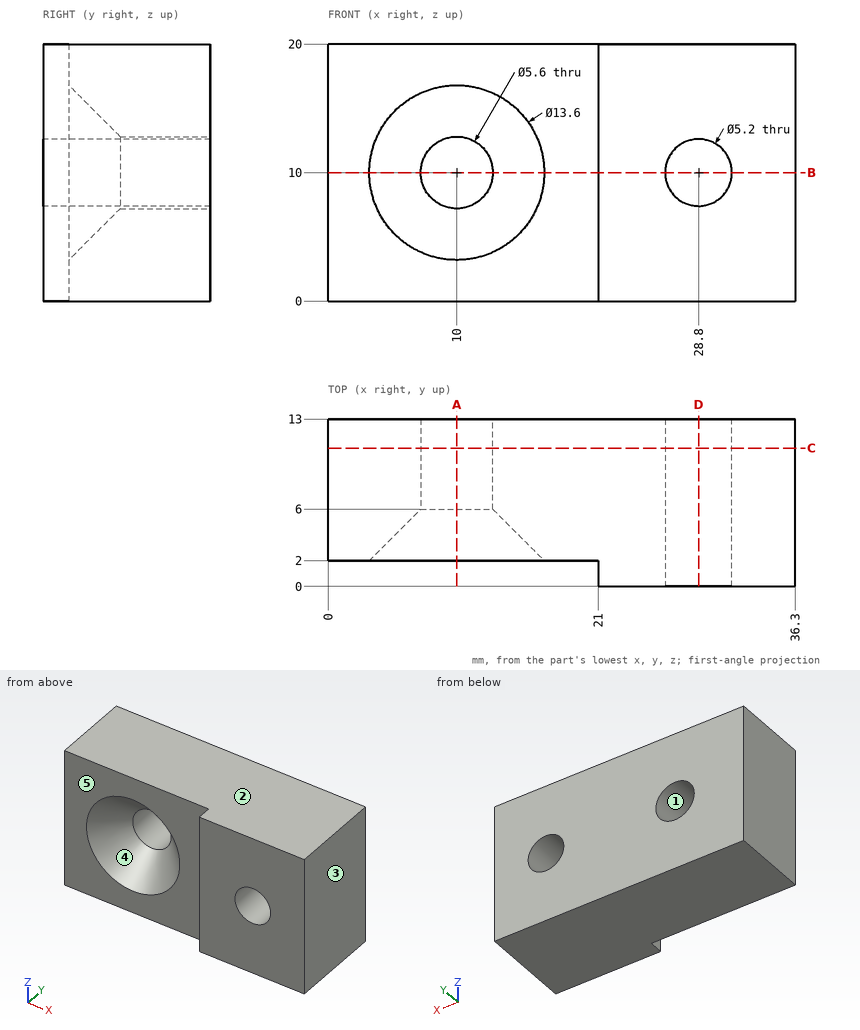
Geometry check sheet. Reference: drawing and pictorial views, mm from the part's lowest x, y, z. A direction names the side the tool comes from. Coordinates: 2 decimals unless noted, no trailing zeros. Order: outer loops, then holes, each group sorted by start corner. A loop starts at its lowest first (then second) coordinate and runs counter-clockwise, first axis right, second up. Notation, with made-up numbers: (1.5, 82.5) -> (21.5, 82.5) arc R22 cw to (21.5, 109.5) -> close; hole circle Ø2 at (54, 53.25). An arc over 180 degrees is marked (long way). Put each result on its own line as item: value. Start each with the question number.
1) Cross-section at D-D (x = 28.8). Enter the section's corners in (y, z).
2) Cross-section at A-A (x = 10). Enter the section's corners in (y, z), plus the area to 3 significant figures.
3) Tool access check on the marked faces 4 and 5. Record the directions out of +Z, -Z, +X, -X, +Y, -Y that give a thin tool (end or side, any length) a straight path to the whole face; none if there is none.
4) Go/stop test with a flat-tipped pin: pin 1 (1.5 mm diameter, centred on y = 6.5, z = 17, fed in from -X). Record where the tip stops, or that it passes through.
5) Cross-section at C-C (y = 10.75). Enter the section's corners in (x, z).
6) Material ranges on L1, parallel to Z at x = 10, y = 10; L2, parallel to Z at x = 28.8, y = 4; L3, parallel to X at y = 0.75, z = 14, recorded low to high.
7) Release check for a two-part mould opening along Z. For the marked faces 1, 2 and 3 record: pulls with the +Z half, pulls with the -Z half, needs draft (parallel to the pull), parting line crosses it, or undercut.
8) Cross-section at B-B (z = 10). Enter the section's corners in (x, y), plus the area to 3 significant figures.
Geometry check:
1. outline: (0, 0) -> (13, 0) -> (13, 7.4) -> (0, 7.4) -> close; (0, 12.6) -> (13, 12.6) -> (13, 20) -> (0, 20) -> close
2. outline: (2, 0) -> (13, 0) -> (13, 7.2) -> (6, 7.2) -> (2, 3.2) -> close; (2, 16.8) -> (6, 12.8) -> (13, 12.8) -> (13, 20) -> (2, 20) -> close
2. area: 142 mm^2
3. face 4: -Y
3. face 5: +Z, -Z, -X, -Y
4. pin 1: stops at x = 0
5. outline: (0, 0) -> (36.3, 0) -> (36.3, 20) -> (0, 20) -> close; hole circle Ø5.6 at (10, 10); hole circle Ø5.2 at (28.8, 10)
6. L1: z = 0 to 7.2, 12.8 to 20
6. L2: z = 0 to 7.4, 12.6 to 20
6. L3: x = 21 to 36.3
7. face 1: undercut
7. face 2: pulls with the +Z half
7. face 3: needs draft
8. outline: (0, 2) -> (3.2, 2) -> (7.2, 6) -> (7.2, 13) -> (0, 13) -> close; (12.8, 6) -> (16.8, 2) -> (21, 2) -> (21, 0) -> (26.2, 0) -> (26.2, 13) -> (12.8, 13) -> close; (31.4, 0) -> (36.3, 0) -> (36.3, 13) -> (31.4, 13) -> close
8. area: 285 mm^2
